from build123d import *

# Parameters (mm, degrees)
EXTRUDE_1_DEPTH             = 35
HOLE_WIZARD_M3_1_AT_2_COUNT = 2
HOLE_WIZARD_M3_1_AT_2_PITCH = 15


with BuildPart() as part:
    # 草圖1 → 填料-伸長1 (new body)
    with BuildSketch(Plane(origin=(0, 35, 0), x_dir=(1, 0, 0), z_dir=(0, 1, 0))):
        with BuildLine():
            Line((8.333333333, 20), (-7.442946108, 10.891560818))
            ThreePointArc((-7.442946108, 10.891560818), (-8.840723587, 9.069941742), (-8.54102232, 6.793484606))
            Line((-8.54102232, 6.793484606), (-3.175426481, -2.5))
            ThreePointArc((-3.175426481, -2.5), (-2.077350269, -3.598076211), (-0.577350269, -4))
            Line((-0.577350269, -4), (50.577350269, -4))
            ThreePointArc((50.577350269, -4), (52.077350269, -3.598076211), (53.175426481, -2.5))
            Line((53.175426481, -2.5), (58.54102232, 6.793484606))
            ThreePointArc((58.54102232, 6.793484606), (58.840723587, 9.069941742), (57.442946108, 10.891560818))
            Line((57.442946108, 10.891560818), (41.666666667, 20))
            Line((41.666666667, 20), (8.333333333, 20))
        make_face()
    extrude(amount=-EXTRUDE_1_DEPTH)

    # 草圖2 → M3 平頭機械螺釘的錐孔1 (revolve, cut)
    with BuildSketch(Plane(origin=(17.5, 0, -8), x_dir=(0, 0, -1), z_dir=(1, 0, 0))):
        Polygon((0, 0), (0, 35), (1.6, 35), (1.6, 28.7), (3.3, 27), (3.3, 0), align=None)
    hole_wizard_m3_1 = revolve(axis=Axis((17.5, -6.35, -8), (0, 1, 0)), mode=Mode.SUBTRACT)

    # M3 平頭機械螺釘的錐孔1 at 2: M3 平頭機械螺釘的錐孔1 ×2
    with Locations(*[(i * HOLE_WIZARD_M3_1_AT_2_PITCH, 0, 0) for i in range(1, HOLE_WIZARD_M3_1_AT_2_COUNT)]):
        add(hole_wizard_m3_1, mode=Mode.SUBTRACT)


solid = part.part
Model file for the job. Use its own axes, mm. A direction names the side the tool comes from. Round coordinates to 2 decimals unless told otherwise and drop trailing zeros. Order: outer loops, then holes, each group sorted by start corner. A loop starts at its lowest first (then second) coordinate and runs counter-clockwise, first axis right, second up. Notation, with made-up numbers: M 7,85.5 L 45,85.5 A10 ccw 45,102.5 Z; hole C -20.75,44 d7. An arc over 180 degrees is marked long. Write each question's results on one line, items separated by ' | '. Start each with the question number.
(1) Two-plate mould, pull along Z, no slides. Class faces 1 (the face through (15.914, 31.806, -7.792)), 2 (the face through (58.85, 17.74, -9.04)), 3 (the face through (25, 35, -8)): pulls with the +Z half, pulls with the -Z half, needs draft (parallel to the pull), parting line crosses it, or undercut.
(2) Drop flat-ended pins along their axis: pin 1 (1 mm diameter, centred on y = 26.5, z = -16, fed in from +X); pin 2 (1 mm diameter, centred on y = 4, z = -15, fed in from +X); pin 3 (5.5 mm diameter, centred on x = 32.5, z = -8, fed in from -Y). Give the stop position or say it passes through.
(3) Saw through at B-B, the plane x = 32.5. Give the cut face in (y, z), then the cut area to 3 significant figures.
(4) Saw through at D-D, the plane x = 1. Give the cut face in (y, z), then the cut area to 3 significant figures.
(5) Probe probe 1 along X at (y, z) = (33.5, -8); probe 2 along X at (y, z) = (14.25, -8); probe 3 along Z at (x, y) = (17.5, 16). List the from-to ranges inside material, lowest first. Write a range as from..to.
(6) Saw through at C-C, the plane z = -8. Give the cut face in (x, y).
(7) Which spindle directions (+Z, -Z, +X, -X, +Y, -Y) get a long thin tool onto all of the face, cutting with end or side? Do faces 4 (the face through (15.27, 13.31, -5.57)), 5 (the face through (0.56, 17.74, -15.51)). Say none if no direction does.
(8) Saw through at A-A, the plane y = 6. Give the cut face in (x, z), then the cut area to 3 significant figures.
Established:
1) face 1: undercut | face 2: parting line crosses it | face 3: needs draft
2) pin 1: stops at x = 49.46 | pin 2: stops at x = 51.19 | pin 3: stops at y = 27.55
3) outline: M 0,-20 L 35,-20 L 35,-9.6 L 28.7,-9.6 L 27,-11.3 L 0,-11.3 Z; M 0,-4.7 L 27,-4.7 L 28.7,-6.4 L 35,-6.4 L 35,4 L 0,4 Z | area: 633 mm^2
4) outline: M 0,-15.77 L 35,-15.77 L 35,4 L 0,4 Z | area: 692 mm^2
5) probe 1: x = -8.93..15.9, 19.1..30.9, 34.1..58.93 | probe 2: x = -8.93..14.2, 20.8..29.2, 35.8..58.93 | probe 3: z = -20..-11.3, -4.7..4
6) outline: M -8.93,0 L 14.2,0 L 14.2,27 L 15.9,28.7 L 15.9,35 L -8.93,35 Z; M 19.1,28.7 L 20.8,27 L 20.8,0 L 29.2,0 L 29.2,27 L 30.9,28.7 L 30.9,35 L 19.1,35 Z; M 34.1,28.7 L 35.8,27 L 35.8,0 L 58.93,0 L 58.93,35 L 34.1,35 Z
7) face 4: -Y | face 5: -Z, -X, +Y, -Y
8) outline: M -8.54,-6.79 A3 ccw -7.44,-10.89 L 8.33,-20 L 41.67,-20 L 57.44,-10.89 A3 ccw 58.54,-6.79 L 53.18,2.5 A3 ccw 50.58,4 L -0.58,4 A3 ccw -3.18,2.5 Z; hole C 17.5,-8 d6.6; hole C 32.5,-8 d6.6 | area: 1,310 mm^2
